from build123d import *

# Parameters (mm, degrees)
SKETCH_1_R             = 20
EXTRUDE_3_DEPTH        = 5
SKETCH_5_R             = 15
EXTRUDE_4_DEPTH        = 80
PATTERN_LINEAR_2_COUNT = 2
PATTERN_LINEAR_2_PITCH = 85


with BuildPart() as part:
    # 草图1 → 凸台-拉伸3 (new body)
    with BuildSketch(Plane.XY):
        with BuildLine():
            Line((-21.594339623, 30), (178.405660377, 30))
            ThreePointArc((178.405660377, 30), (208.405660377, 0), (178.405660377, -30))
            Line((178.405660377, -30), (-21.594339623, -30))
            ThreePointArc((-21.594339623, -30), (-51.594339623, 0), (-21.594339623, 30))
        make_face()
        with Locations((178.405660377, 0)):
            Circle(SKETCH_1_R, mode=Mode.SUBTRACT)
        with Locations((-21.594339623, 0)):
            Circle(SKETCH_1_R, mode=Mode.SUBTRACT)
    extrude_3 = extrude(amount=EXTRUDE_3_DEPTH)

    # 草图5 → 凸台-拉伸4 (add)
    with BuildSketch(Plane.XY.offset(5)):
        with Locations((37.971935237, 0)):
            Circle(SKETCH_5_R)
        with Locations((108.550446531, 0)):
            Circle(SKETCH_5_R)
    extrude(amount=EXTRUDE_4_DEPTH)

    # 阵列(线性)2: 凸台-拉伸3 ×2
    with Locations(*[(0, 0, i * PATTERN_LINEAR_2_PITCH) for i in range(1, PATTERN_LINEAR_2_COUNT)]):
        add(extrude_3)


solid = part.part
Build history of the part. All positions in model axes, mm. A direction names the side the tool comes from. Give positions to 0.01 mm unless a question says otherwise; leave off trailing zeros. Loops run counter-clockwise (first coordinate to the right, second up) from the corner with the lowest first, then second, coordinate; pieces in that order, holes last. Notation, with made-up numbers: (7, -20.5) - (41, -20.5) arc R21 ccw to (41, -2.5) - close; hole circle Ø5 at (48, 37.25). An arc over 180 degrees is marked (long way). Write item = value, one per line. Start each with the question number.
1) Drop flat-ended pins along their axis: pin 1 Ø1 at (y, z) = (10, 21.5) entering from -X; pin 2 Ø8 at (y, z) = (-12, 59.5) entering from +X; pin 3 Ø1.5 at (y, z) = (12.5, 35.5) entering from -X. Give the stop position or say it passes through.
2) Pull direction Y, two halves, no side cores. Call faces 1 (the cylindrical face through (-51.587, -0.66, 87.465)), 2 (the cylindrical face through (-2.52, 6.01, 87.46)), 3 (the flat face through (80, 0, 85)): +Y half, -Y half, draft (parallel to the pull), parting line (faces both ways), or undercut.
3) Band-saw the part on C-C on y = -26. Give the cut face in (x, z), plus the area to 3 significant figures.
4) Band-saw the part on D-D on z = 68. Give the cut face in (x, y), plus the area to 3 significant figures.
5) Band-saw the part on B-B on x = 144.5. Give the cut face in (y, z).
6) Band-saw the part on A-A on y = 0. Count the separate pieces of the cut face and the enclosed holes in it, plus the area to 3 significant figures.
7) Tool access for faces 4 (the cylindrical face through (122.858, 4.506, 44.44)), 5 (the cylindrical face through (-2.52, 6.01, 2.46)): list every direction of +Z, -Z, +X, -X, +Y, -Y with a clear straight run to the whole face (end or side of a thin tool).
8) Probe probe 1 along X at (y, z) = (-1, 39); probe 2 along Z at (x, y) = (111, -16.5); probe 3 along X at (y, z) = (12, 62). List the from-to ranges inside material, lowest first. Write a range as from..to.
Final values:
q1.pin_1 = 26.36
q1.pin_2 = 121.24
q1.pin_3 = 28.65
q2.face_1 = parting line
q2.face_2 = undercut
q2.face_3 = draft
q3.outline = (-36.56, 0) - (193.37, 0) - (193.37, 5) - (-36.56, 5) - close; (-36.56, 85) - (193.37, 85) - (193.37, 90) - (-36.56, 90) - close
q3.area = 2,300 mm²
q4.outline = circle Ø30 at (37.97, 0); circle Ø30 at (108.55, 0)
q4.area = 1,410 mm²
q5.outline = (-30, 0) - (30, 0) - (30, 5) - (-30, 5) - close; (-30, 85) - (30, 85) - (30, 90) - (-30, 90) - close
q6.separate_pieces = 5
q6.enclosed_holes = 1
q6.area = 6,600 mm²
q7.face_4 = none
q7.face_5 = +Z, -Z
q8.probe_1 = 23.01..52.94, 93.58..123.52
q8.probe_2 = 0..5, 85..90
q8.probe_3 = 28.97..46.97, 99.55..117.55
